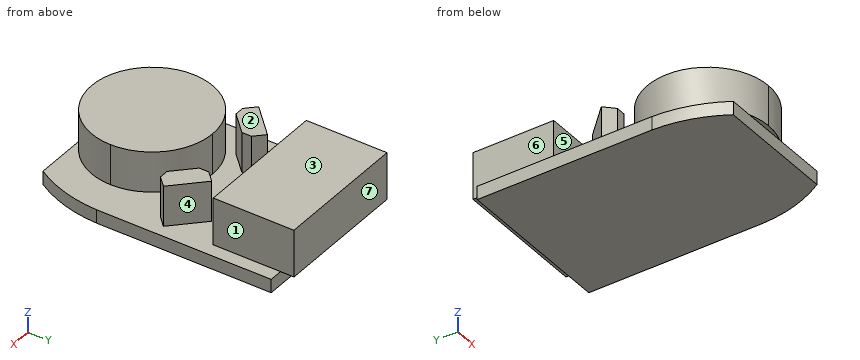
from build123d import *

# Parameters (mm, degrees)
BOSS_EXTRU_1_DEPTH = 1
BOSS_EXTRU_2_START = 1
BOSS_EXTRU_2_DEPTH = 1
BOSS_EXTRU_3_START = 2
BOSS_EXTRU_3_DEPTH = 3
BOSS_EXTRU_4_START = 1
ESQUISSE1_6_W      = 10
ESQUISSE1_6_H      = 6
BOSS_EXTRU_4_DEPTH = 3.5
BOSS_EXTRU_5_DEPTH = 3


with BuildPart() as part:
    # Esquisse1 → Boss.-Extru.1 (new body)
    with BuildSketch(Plane.XY):
        with BuildLine():
            Line((-6, 0), (-6, 13))
            Line((-6, 13), (6, 13))
            Line((6, 13), (6, 0))
            ThreePointArc((6, 0), (5.582013923, -2.599604177), (4.5, -5))
            Line((4.5, -5), (-4.5, -5))
            ThreePointArc((-4.5, -5), (-5.582013923, -2.599604177), (-6, 0))
        make_face()
    extrude(amount=BOSS_EXTRU_1_DEPTH)

    # Esquisse1<4> → Boss.-Extru.2 (add)
    with BuildSketch(Plane.XY.offset(BOSS_EXTRU_2_START)):
        with BuildLine():
            ThreePointArc((0, 0.5), (-0.5, 0), (0, -0.5))
            Line((0, -0.5), (0, 0.5))
        make_face()
        with BuildLine():
            Line((0, 0.5), (0, -0.5))
            ThreePointArc((0, -0.5), (0.353553391, -0.353553391), (0.5, 0))
            ThreePointArc((0.5, 0), (0.353553391, 0.353553391), (0, 0.5))
        make_face()
    extrude(amount=BOSS_EXTRU_2_DEPTH)

    # Esquisse1<5> → Boss.-Extru.3 (add)
    with BuildSketch(Plane.XY.offset(BOSS_EXTRU_3_START)):
        with BuildLine():
            ThreePointArc((0, 4.5), (-4.5, 0), (0, -4.5))
            Line((0, -4.5), (0, -0.5))
            ThreePointArc((0, -0.5), (-0.5, 0), (0, 0.5))
            Line((0, 0.5), (0, 4.5))
        make_face()
        with BuildLine():
            Line((0, -0.5), (0, -4.5))
            ThreePointArc((0, -4.5), (3.181980515, -3.181980515), (4.5, 0))
            ThreePointArc((4.5, 0), (3.181980515, 3.181980515), (0, 4.5))
            Line((0, 4.5), (0, 0.5))
            ThreePointArc((0, 0.5), (0.353553391, 0.353553391), (0.5, 0))
            ThreePointArc((0.5, 0), (0.353553391, -0.353553391), (0, -0.5))
        make_face()
        with BuildLine():
            ThreePointArc((0, 0.5), (-0.5, 0), (0, -0.5))
            Line((0, -0.5), (0, 0.5))
        make_face()
        with BuildLine():
            Line((0, 0.5), (0, -0.5))
            ThreePointArc((0, -0.5), (0.353553391, -0.353553391), (0.5, 0))
            ThreePointArc((0.5, 0), (0.353553391, 0.353553391), (0, 0.5))
        make_face()
    extrude(amount=BOSS_EXTRU_3_DEPTH)

    # Esquisse1<6> → Boss.-Extru.4 (add)
    with BuildSketch(Plane.XY.offset(BOSS_EXTRU_4_START)):
        with Locations((0, 11)):
            Rectangle(ESQUISSE1_6_W, ESQUISSE1_6_H)
    extrude(amount=BOSS_EXTRU_4_DEPTH)

    # Esquisse2 → Boss.-Extru.5 (add)
    with BuildSketch(Plane.XY.offset(1)):
        Polygon((-5.121320344, 4.378679656), (-3, 6.5), (-2.292893219, 5.792893219), (-2.292893219, 5.085786438), (-3.707106781, 3.671572875), (-4.414213562, 3.671572875), align=None)
    boss_extru_5 = extrude(amount=BOSS_EXTRU_5_DEPTH)

    # Symétrie1: Boss.-Extru.5 across plane
    add(boss_extru_5.mirror(Plane(origin=(0, 0, 0), x_dir=(0, 0, 1), z_dir=(1, 0, 0))))


solid = part.part
Input: part model. Units: mm. Frame: model coordinates. Face numbers are marked on the shaded views. A direction names the side the tool comes from. Give positions to 0.01 mm unless a question says otherwise; leave off trailing zeros. Write each loop counter-clockwise with the first axis right and the second up, starting at its lowest first coordinate (ties: lowest second). Pieces come first, ordered by that corner, then holes. Notation, with made-up numbers: M 75,85 L 120,85 A15 ccw 120,93 Z; hole C 70.25,9.5 d3. An arc over 180 degrees is marked long. Write item = value, one per line. Start each with the question number.
1) Reachability of the marked faces 1, 2 and 3 from +Z, -Z, +X, -X, +Y, -Y: full face, straight path, thin tool, end or side. Return the list, or none.
2) Cut plane B-B on z = 4.2. Return the cut outline in (x, y).
3) Cut plane A-A on z = 2.65. Return the cut outline in (x, y), then the cut area to 3 significant figures.
4) Draft query along Y for the marked faces 4, 5, 6 and 7. Return one class per face: +Y half, -Y half, draft (parallel to the pull), parting line (faces both ways), or undercut.
5) First-contact query: pin 1 Ø0.6 at (y, z) = (5.5, 2.5) entering from +X; pin 2 Ø3 at (y, z) = (5, 3.5) entering from -X; pin 3 Ø3 at (x, y) = (-0.5, 10) entering from +Z. Flat tips, straight axial feed; report the tip coordinate or a pass-through.
6) Cut plane C-C on x = 3.25. Return the cut outline in (y, z), then the cut area to 3 significant figures.
7) Material intervals for line 1 along Z through (x, y) = (-1.75, -4); line 2 along Y through (x, z) = (-4, 3.45); line 3 along Y through (x, z) = (3.25, 2.85), sorted ascending. Write a range as [from, to].
8) Cut plane D-D on y = 1.5. Return the cut outline in (x, z), then the cut area to 3 significant figures.
Solved:
q1.face_1 = +Z, +X, +Y
q1.face_2 = +Z, -X
q1.face_3 = +Z, +X, -X, +Y
q2.outline = M -5,8 L 5,8 L 5,14 L -5,14 Z; C 0,0 d9
q3.outline = M -5.12,4.38 L -4.41,3.67 L -3.71,3.67 L -2.29,5.09 L -2.29,5.79 L -3,6.5 Z; M -5,8 L 5,8 L 5,14 L -5,14 Z; C 0,0 d9; M 2.29,5.09 L 3.71,3.67 L 4.41,3.67 L 5.12,4.38 L 3,6.5 L 2.29,5.79 Z
q3.area = 132 mm2
q4.face_4 = undercut
q4.face_5 = undercut
q4.face_6 = draft
q4.face_7 = +Y half
q5.pin_1 = 4.3
q5.pin_2 = -5.12
q5.pin_3 = 4.5
q6.outline = M -5,0 L 13,0 L 13,1 L 14,1 L 14,4.5 L 8,4.5 L 8,1 L 6.25,1 L 6.25,4 L 4.13,4 L 4.13,1 L -5,1 Z; M -3.11,2 L 3.11,2 L 3.11,5 L -3.11,5 Z
q6.area = 64.0 mm2
q7.line_1 = [0, 1], [2, 5]
q7.line_2 = [-2.06, 2.06], [3.67, 5.5], [8, 14]
q7.line_3 = [-3.11, 3.11], [4.13, 6.25], [8, 14]
q8.outline = M -6,0 L 6,0 L 6,1 L -6,1 Z; M -4.24,2 L 4.24,2 L 4.24,5 L -4.24,5 Z
q8.area = 37.5 mm2
